The drawing under review shows one solid part. Ordinate dimensions are in mm from its lowest x, y, z. Coordinates: 2 decimals unless noted, no trailing zeros. Write each loop counter-clockwise with the first axis right and the second up, starting at its lowest first coordinate (ties: lowest second). Pieces come first, ordered by that corner, then holes. Notation, with made-up numbers: M 61.25,18 L 110.25,18 A28 ccw 110.25,44 Z; hole C -23,-24.75 d8. An arc over 180 degrees is marked long. Write each question's results on one line, items separated by ' | '. Start each with the question number.
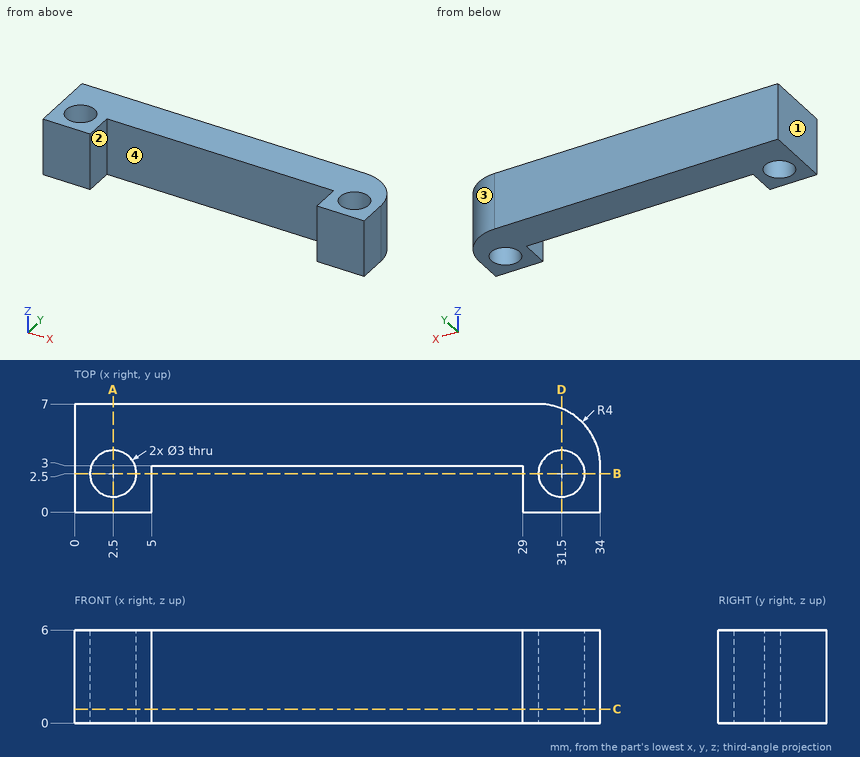
Item 1: Draft analysis for pull direction X (two halves, no side actions). For the marked faces 1, 2, 3 and 4, state which applies: released by +X, released by -X, zero draft, split by the parting line, or undercut.
Item 2: Wall thickness on L1, parallel to Y at x = 2.5, z = 1.8; L2, parallel to Y at x = 11.5, z = 4.25; L3, parallel to X at y = 2.25, z = 3.85: over which ranges is each line inside the solid? List them lowest first.
Item 3: We need section C-C on z = 0.9. State the section outline as (x, y) points, then the cut area to 3 significant figures.
Item 4: Insertion check: pin 1 Ø1 at (x, z) = (14.5, 3) entering from -Y. The pin has a flat end and moves straight along its axis. Give the tip position at first contact, or say it passes through.
Item 5: We need section D-D on x = 31.5. State the section outline as (y, z) points.
Item 6: We need section B-B on y = 2.5. State the section outline as (x, z) points, then the cut area to 3 significant figures.
Item 7: We need section A-A on x = 2.5. State the section outline as (y, z) points.
Answer:
1) face 1: released by -X | face 2: undercut | face 3: released by +X | face 4: undercut
2) L1: y = 0 to 1, 4 to 7 | L2: y = 3 to 7 | L3: x = 0 to 1.02, 3.98 to 5, 29 to 30.02, 32.98 to 34
3) outline: M 0,0 L 5,0 L 5,3 L 29,3 L 29,0 L 34,0 L 34,3 A4 ccw 30,7 L 0,7 Z; hole C 2.5,2.5 d3; hole C 31.5,2.5 d3 | area: 148 mm^2
4) pin 1: stops at y = 3
5) outline: M 0,0 L 1,0 L 1,6 L 0,6 Z; M 4,0 L 6.71,0 L 6.71,6 L 4,6 Z
6) outline: M 0,0 L 1,0 L 1,6 L 0,6 Z; M 4,0 L 5,0 L 5,6 L 4,6 Z; M 29,0 L 30,0 L 30,6 L 29,6 Z; M 33,0 L 34,0 L 34,6 L 33,6 Z | area: 24.0 mm^2
7) outline: M 0,0 L 1,0 L 1,6 L 0,6 Z; M 4,0 L 7,0 L 7,6 L 4,6 Z
